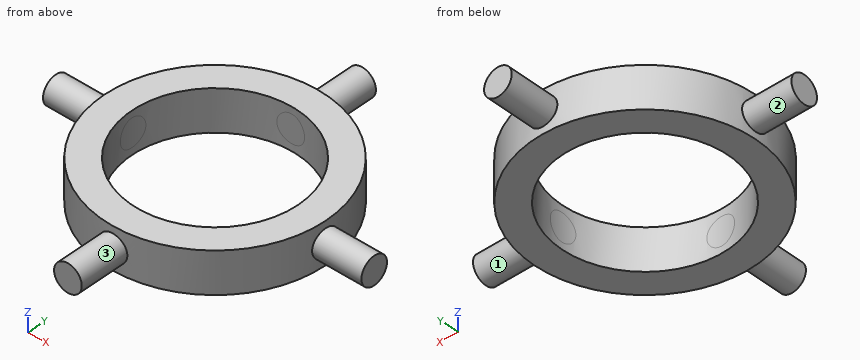
from build123d import *

# Parameters (mm, degrees)
CROQUIS2_R              = 40
CROQUIS2_R_2            = 30
SALIENTE_EXTRUIR1_DEPTH = 7.5
CROQUIS3_R              = 5
SALIENTE_EXTRUIR2_DEPTH = 57.5
CROQUIS4_R              = 5
SALIENTE_EXTRUIR3_DEPTH = 57.5
CORTAR_EXTRUIR1_START   = -115
CROQUIS5_R              = 30
CORTAR_EXTRUIR1_DEPTH   = 115


with BuildPart() as part:
    # Croquis2 → Saliente-Extruir1 (new, symmetric)
    with BuildSketch(Plane.XY):
        Circle(CROQUIS2_R)
        Circle(CROQUIS2_R_2, mode=Mode.SUBTRACT)
    extrude(amount=SALIENTE_EXTRUIR1_DEPTH, both=True)

    # Croquis3 → Saliente-Extruir2 (add, symmetric)
    with BuildSketch(Plane(origin=(0, 0, 0), x_dir=(1, 0, 0), z_dir=(0, 1, 0))):
        with Locations(Location((0, 0, 0), (0, 0, 90))):
            Circle(CROQUIS3_R)
    extrude(amount=SALIENTE_EXTRUIR2_DEPTH, both=True)

    # Croquis4 → Saliente-Extruir3 (add, symmetric)
    with BuildSketch(Plane(origin=(0, 0, 0), x_dir=(0, 0, -1), z_dir=(1, 0, 0))):
        with Locations(Location((0, 0, 0), (0, 0, 180))):
            Circle(CROQUIS4_R)
    extrude(amount=SALIENTE_EXTRUIR3_DEPTH, both=True)

    # Croquis5 → Cortar-Extruir1 (cut)
    with BuildSketch(Plane.XY.offset(7.5).offset(CORTAR_EXTRUIR1_START)):
        Circle(CROQUIS5_R)
    extrude(amount=CORTAR_EXTRUIR1_DEPTH, mode=Mode.SUBTRACT)


solid = part.part
Design review of the part built by this model. Coordinates are the model's own, in mm. Face numbers are marked on the shaded views. A direction names the side the tool comes from. Round coordinates to 2 decimals unless told otherwise and drop trailing zeros. Loops run counter-clockwise (first coordinate to the right, second up) from the corner with the lowest first, then second, coordinate; pieces in that order, holes last. Notation, with made-up numbers: (44, 48) -> (90, 48) arc R22 cw to (90, 73) -> close; hole circle Ø11 at (69, -15). An arc over 180 degrees is marked (long way). Use one line per item in the form item = value. Start each with the question number.
Q1. We need section D-D on y = 49.5. Give the boundary of the cut face in (x, z).
Q2. Machinability: for the marked faces 1, 2 and 3, which of the approach directions +Z, -Z, +X, -X, +Y, -Y give a long, thin tool a straight path to every point of the face, cutting with its end or side? Answer none if there is none.
Q3. For pin 1 Ø6 at (y, z) = (-31.5, -5.5) entering from -X; pin 2 Ø1 at (y, z) = (6, -2) entering from +X; pin 3 Ø3 at (x, z) = (37.5, -0.5) entering from +Y; pin 4 Ø3 at (x, y) = (40.5, 1) entering from -Z, all flat-tipped, find the tip position at first contact; note any pin that passes through.
Q4. We need section A-A on x = -10.5. Give the boundary of the cut face in (y, z), then the cut area to 3 significant figures.
Q5. We need section B-B on y = -3. Give the boundary of the cut face in (x, z).
Q6. We need section C-C on z = 3.5. Give the boundary of the cut face in (x, y).
Q7. Wall thickness on line 1 along X through (y, z) = (0, -0.5); line 2 along X through (y, z) = (-17.5, 5): over which ranges is each line inside the solid? List them lowest first. Write a range as [from, to].
Calculated:
q1.outline = circle Ø10 at (0, 0)
q2.face_1 = +X
q2.face_2 = -X
q2.face_3 = -Y
q3.pin_1 = -28.07
q3.pin_2 = 39.62
q3.pin_3 = 17.44
q3.pin_4 = -7.5
q4.outline = (-38.6, -7.5) -> (-28.1, -7.5) -> (-28.1, 7.5) -> (-38.6, 7.5) -> close; (28.1, -7.5) -> (38.6, -7.5) -> (38.6, 7.5) -> (28.1, 7.5) -> close
q4.area = 315 mm²
q5.outline = (-57.5, -4) -> (-39.89, -4) -> (-39.89, -7.5) -> (-29.85, -7.5) -> (-29.85, 7.5) -> (-39.89, 7.5) -> (-39.89, 4) -> (-57.5, 4) -> close; (29.85, -7.5) -> (39.89, -7.5) -> (39.89, -4) -> (57.5, -4) -> (57.5, 4) -> (39.89, 4) -> (39.89, 7.5) -> (29.85, 7.5) -> close
q6.outline = (-57.5, -3.57) -> (-39.84, -3.57) arc R40 ccw to (-3.57, -39.84) -> (-3.57, -57.5) -> (3.57, -57.5) -> (3.57, -39.84) arc R40 ccw to (39.84, -3.57) -> (57.5, -3.57) -> (57.5, 3.57) -> (39.84, 3.57) arc R40 ccw to (3.57, 39.84) -> (3.57, 57.5) -> (-3.57, 57.5) -> (-3.57, 39.84) arc R40 ccw to (-39.84, 3.57) -> (-57.5, 3.57) -> close; hole circle Ø60 at (0, 0)
q7.line_1 = [-57.5, -30], [30, 57.5]
q7.line_2 = [-35.97, -24.37], [24.37, 35.97]
